Design review of the part shown in the three views and the two pictorial views. Dimensions are in mm from the part's minimum x, y and z. Give positions to 0.01 mm unless a question says otherwise; leave off trailing zeros. Write each loop counter-clockwise with the first axis right and the second up, starting at its lowest first coordinate (ties: lowest second). Pieces come first, ordered by that corner, then holes. Notation, with made-up numbers: M 68.25,-37 L 103.25,-37 A29 ccw 103.25,-11 Z; hole C -37,77 d3. An arc over 180 degrees is marked long. Write item = value, one per line.
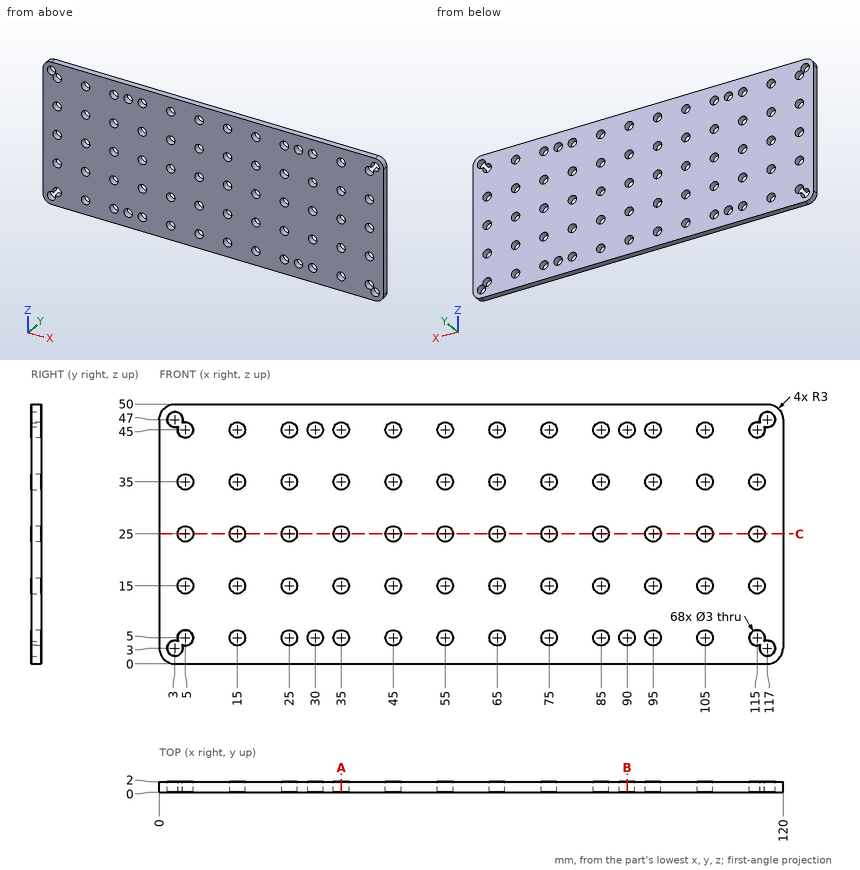
1. We need section A-A, the plane x = 35. Write out the cut boundary in (y, z), then the cut area to 3 significant figures.
Responses:
outline = M 0,0 L 2,0 L 2,3.5 L 0,3.5 Z; M 0,6.5 L 2,6.5 L 2,13.5 L 0,13.5 Z; M 0,16.5 L 2,16.5 L 2,23.5 L 0,23.5 Z; M 0,26.5 L 2,26.5 L 2,33.5 L 0,33.5 Z; M 0,36.5 L 2,36.5 L 2,43.5 L 0,43.5 Z; M 0,46.5 L 2,46.5 L 2,50 L 0,50 Z
area = 70.0 mm2
2. For line 1 along X through (y, z) = (1.5, 47); line 2 along Z through (x, y) = (29, 1.5), list the stretches that pass through material, from the lowest coordinate up. Write a range as from..to.
Responses:
line_1 = 0..1.5, 4.5..115.5, 118.5..120
line_2 = 0..3.88, 6.12..43.88, 46.12..50
3. We need section B-B, the plane x = 90. Write out the cut boundary in (y, z).
Responses:
outline = M 0,0 L 2,0 L 2,3.5 L 0,3.5 Z; M 0,6.5 L 2,6.5 L 2,43.5 L 0,43.5 Z; M 0,46.5 L 2,46.5 L 2,50 L 0,50 Z
4. We need section C-C, the plane z = 25. Count the separate pieces of the cut face and the enclosed holes in it, then the cut area to 3 significant figures.
Responses:
separate_pieces = 13
enclosed_holes = 0
area = 168 mm2
